from build123d import *

# Parameters (mm, degrees)
SKETCH1_W           = 12
SKETCH1_H           = 12
BOSS_EXTRUDE1_DEPTH = 6.5
SKETCH5_W           = 1.6
SKETCH5_H           = 0.4
BOSS_EXTRUDE3_DEPTH = 0.5
SKETCH6_W           = 1.6
SKETCH6_H           = 0.4
BOSS_EXTRUDE4_DEPTH = 0.4
FILLET1_R           = 0.6
FILLET2_R           = 0.3


with BuildPart() as part:
    # Sketch1 → Boss-Extrude1 (new body)
    with BuildSketch(Plane.XY):
        with Locations((6, 6)):
            Rectangle(SKETCH1_W, SKETCH1_H)
    extrude(amount=BOSS_EXTRUDE1_DEPTH)

    # Sketch4 → Revolve1 (revolve)
    with BuildSketch(Plane(origin=(0, 6, 0), x_dir=(1, 0, 0), z_dir=(0, 1, 0))):
        with BuildLine():
            Line((3.35, -8.6), (3.35, -6.5))
            Line((3.35, -6.5), (6, -6.5))
            Line((6, -6.5), (6, -9.1))
            ThreePointArc((6, -9.1), (4.643872087, -9.014977939), (3.35, -8.6))
        make_face()
    revolve(axis=Axis((6, 6, 6.5), (0, 0, 1)))

    # Sketch5 → Boss-Extrude3 (add)
    with BuildSketch(Plane.XZ):
        with Locations((8.65, 3.4)):
            Rectangle(SKETCH5_W, SKETCH5_H)
        with Locations((3.35, 3.4)):
            Rectangle(SKETCH5_W, SKETCH5_H)
    extrude(amount=BOSS_EXTRUDE3_DEPTH)

    # Sketch6 → Boss-Extrude4 (add)
    with BuildSketch(Plane.XZ.offset(0.5)):
        with BuildLine():
            Line((2.95, 0), (2.95, -1.9))
            ThreePointArc((2.95, -1.9), (3.35, -2.2), (3.75, -1.9))
            Line((3.75, -1.9), (3.75, 0))
            Line((3.75, 0), (4.15, 0.4))
            Line((4.15, 0.4), (4.15, 3.2))
            Line((4.15, 3.2), (2.55, 3.2))
            Line((2.55, 3.2), (2.55, 0.4))
            Line((2.55, 0.4), (2.95, 0))
        make_face()
        with Locations((3.35, 3.4)):
            Rectangle(SKETCH6_W, SKETCH6_H)
        with BuildLine():
            ThreePointArc((9.05, -1.9), (8.65, -2.2), (8.25, -1.9))
            Line((8.25, -1.9), (8.25, 0))
            Line((8.25, 0), (7.85, 0.4))
            Line((7.85, 0.4), (7.85, 3.6))
            Line((7.85, 3.6), (9.45, 3.6))
            Line((9.45, 3.6), (9.45, 0.4))
            Line((9.45, 0.4), (9.05, 0))
            Line((9.05, 0), (9.05, -1.9))
        make_face()
    extrude(amount=BOSS_EXTRUDE4_DEPTH)

    # Fillet1
    fillet1_edges = [part.edges().sort_by_distance(p)[0] for p in [
        (3.35, -0.9, 3.6),
        (8.65, -0.9, 3.6),
    ]]
    fillet(fillet1_edges, radius=FILLET1_R)

    # Fillet2
    fillet2_edges = [part.edges().sort_by_distance(p)[0] for p in [
        (3.35, -0.5, 3.2),
        (8.65, -0.5, 3.2),
    ]]
    fillet(fillet2_edges, radius=FILLET2_R)


solid = part.part
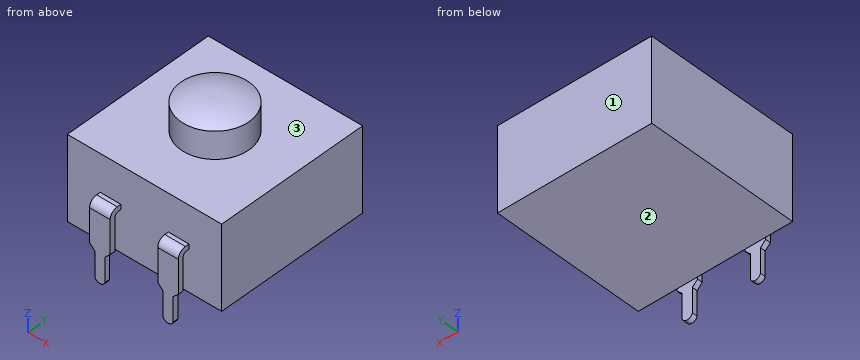
For this review, take the finished solid that the model builds, in its own axes (mm). Face numbers are marked on the shaded views. A direction names the side the tool comes from. Give positions to 0.01 mm unless a question says otherwise; leave off trailing zeros. Order: outer loops, then holes, each group sorted by start corner. A loop starts at its lowest first (then second) coordinate and runs counter-clockwise, first axis right, second up. Notation, with made-up numbers: M 78.25,-36 L 97.25,-36 A22 cw 97.25,-1 Z; hole C -10,68.25 d8. An arc over 180 degrees is marked long. Answer in a Markdown table with one row per item. Add a question column.
(1) Wall thickness on probe 1 along Y at (x, z) = (8.5, 1.5); probe 2 along Y at (x, z) = (5.75, 0.25); probe 3 along Z at (x, y) = (5.5, 9.25): over which ranges is each line inside the solid? List them lowest first. Write a range as [from, to].
(2) Consider section B-B on z = 1. State the section outline as (x, y) points.
(3) For the marked faces 1, 2 and 3, list the 3-axis set-ups (+Z, -Z, +X, -X, +Y, -Y) from which the entire face can be reached by the end or side of a thin tool; tool diameter is ignored.
(4) Consider section C-C on x = 10. State the section outline as (y, z) points.
(5) For pin 1 (3.5 mm diameter, centred on x = 7.5, y = 7, fed in from -Z); pin 2 (3 mm diameter, centred on x = 10.5, y = 3.5, fed in from +Z); pin 3 (0.5 mm diameter, centred on x = 3.5, z = -0.5, fed in from +Y), all flat-tipped, find the tip position at first contact; note any pin that passes through.
(6) Consider section A-A on z = -1.25. State the section outline as (x, y) points.
Evaluation:
| question | item | result |
|---|---|---|
| 1 | probe 1 | y = [-0.9, -0.5], [0, 12] |
| 1 | probe 2 | y = [0, 12] |
| 1 | probe 3 | z = [0, 6.5] |
| 2 | outline | M 0,0 L 12,0 L 12,12 L 0,12 Z; M 2.55,-0.9 L 4.15,-0.9 L 4.15,-0.5 L 2.55,-0.5 Z; M 7.85,-0.9 L 9.45,-0.9 L 9.45,-0.5 L 7.85,-0.5 Z |
| 3 | face 1 | +Z, -Z, +X, -X, +Y |
| 3 | face 2 | -Z, +X, -X, +Y |
| 3 | face 3 | +Z |
| 4 | outline | M 0,0 L 12,0 L 12,6.5 L 0,6.5 Z |
| 5 | pin 1 | stops at z = 0 |
| 5 | pin 2 | stops at z = 6.5 |
| 5 | pin 3 | stops at y = -0.5 |
| 6 | outline | M 2.95,-0.9 L 3.75,-0.9 L 3.75,-0.5 L 2.95,-0.5 Z; M 8.25,-0.9 L 9.05,-0.9 L 9.05,-0.5 L 8.25,-0.5 Z |
